The listing builds one solid part. Answer for the finished solid, in the listing's coordinates (mm). A direction names the side the tool comes from. Give positions to 0.01 mm unless a question says otherwise; leave off trailing zeros. Write each loop counter-clockwise with the first axis right and the second up, starting at its lowest first coordinate (ties: lowest second). Pieces come first, ordered by that corner, then holes. Notation, with made-up numbers: (43.5, -34) -> (69.5, -34) arc R17 ccw to (69.5, -9) -> close; hole circle Ø6 at (32, -17.5). An arc over 180 degrees is marked (long way). Write each question's results on one line, items separated by ' | '. Start each with the question number.
from build123d import *

# Parameters (mm, degrees)
BOSS_EXTRUDE1_DEPTH = 5
FILLET1_R           = 1
SKETCH2_R           = 1.5
CUT_EXTRUDE1_DEPTH  = 10


with BuildPart() as part:
    # Sketch1 → Boss-Extrude1 (new body, symmetric)
    with BuildSketch(Plane.XY):
        with BuildLine():
            Line((4, 0), (12, 0))
            Line((12, 0), (12, 1))
            Line((12, 1), (4.898979486, 1))
            ThreePointArc((4.898979486, 1), (0, 5), (-4.898979486, 1))
            Line((-4.898979486, 1), (-12, 1))
            Line((-12, 1), (-12, 0))
            Line((-12, 0), (-4, 0))
            ThreePointArc((-4, 0), (0, 4), (4, 0))
        make_face()
    extrude(amount=BOSS_EXTRUDE1_DEPTH, both=True)

    # Fillet1
    fillet1_edges = [part.edges().sort_by_distance(p)[0] for p in [
        (-12, 0.5, -5),
        (-12, 0.5, 5),
        (12, 0.5, 5),
        (12, 0.5, -5),
    ]]
    fillet(fillet1_edges, radius=FILLET1_R)

    # Sketch2 → Cut-Extrude1 (cut)
    with BuildSketch(Plane(origin=(0, 1, 0), x_dir=(1, 0, 0), z_dir=(0, 1, 0))):
        with Locations((-8, 0)):
            Circle(SKETCH2_R)
        with Locations((8, 0)):
            Circle(SKETCH2_R)
    extrude(amount=-CUT_EXTRUDE1_DEPTH, mode=Mode.SUBTRACT)


solid = part.part
1. Section C-C (z = -2) is taken. Write down the section's boundary in (x, y).
2. Section A-A (x = 8) is taken. Write down the section's boundary in (y, z), then the cut area to 3 significant figures.
3. A tool of negligible diameter and unlimited length cuts with its end or side. For faces 1 (the cylindrical face through (11.715, 0.507, -4.699)), 2 (the flat face through (-9.2, 1, 1.2)), from which of +Z, -Z, +X, -X, +Y, -Y can it reach the whole face along a straight path? Write none if from no direction.
4. Consider probe 1 along X at (y, z) = (0.6, 0); probe 2 along Z at (x, y) = (8, 0.3); probe 3 along Y at (x, z) = (6.5, -2.75). Determine where each line is inside the solid, lowest interval first. Write a range as [from, to].
5. Section B-B (y = 2.15) is taken. Write down the section's boundary in (x, z), then the cut area to 3 significant figures.
6. The mould has two halves that part along X. Classify faces 3 (the cylindrical face through (-9.5, 0.51, -0.07)), 4 (the flat face through (9.3, 1, 1.2)), 5 (the cylindrical face through (6.5, 0.51, -0.07)), 6 (the cylindrical face through (0, 5, 0)): pulls with the +X half, pulls with the -X half, needs draft (parallel to the pull), parting line crosses it, or undercut.
7. Section D-D (y = 0.6) is taken. Write down the section's boundary in (x, z), then the cut area to 3 significant figures.
8. Each of these flat-tipped pins is pushed along its axis until it touches: pin 1 Ø3 at (x, z) = (4, -1.5) entering from +Y; pin 2 Ø1 at (x, z) = (-6, 2.5) entering from -Y; pin 3 Ø3 at (x, z) = (5.5, 0.5) entering from +Y; pin 4 Ø1 at (y, z) = (3, -2.5) entering from -X. Where does it stop, or does it pass through?
Results:
1) outline: (-12, 0) -> (-4, 0) arc R4 cw to (4, 0) -> (12, 0) -> (12, 1) -> (4.9, 1) arc R5 ccw to (-4.9, 1) -> (-12, 1) -> close
2) outline: (0, -5) -> (1, -5) -> (1, -1.5) -> (0, -1.5) -> close; (0, 1.5) -> (1, 1.5) -> (1, 5) -> (0, 5) -> close | area: 7.00 mm²
3) face 1: -Z, +X, +Y, -Y | face 2: +Z, -Z, -X, +Y
4) probe 1: x = [-12, -9.5], [-6.5, -3.95], [3.95, 6.5], [9.5, 12] | probe 2: z = [-5, -1.5], [1.5, 5] | probe 3: y = [0, 1]
5) outline: (-4.51, -5) -> (-3.37, -5) -> (-3.37, 5) -> (-4.51, 5) -> close; (3.37, -5) -> (4.51, -5) -> (4.51, 5) -> (3.37, 5) -> close | area: 22.8 mm²
6) face 3: undercut | face 4: needs draft | face 5: undercut | face 6: parting line crosses it
7) outline: (-12, -4) arc R1 ccw to (-11, -5) -> (-3.95, -5) -> (-3.95, 5) -> (-11, 5) arc R1 ccw to (-12, 4) -> close; (3.95, -5) -> (11, -5) arc R1 ccw to (12, -4) -> (12, 4) arc R1 ccw to (11, 5) -> (3.95, 5) -> close; hole circle Ø3 at (-8, 0); hole circle Ø3 at (8, 0) | area: 146 mm²
8) pin 1: stops at y = 4.33 | pin 2: stops at y = 0 | pin 3: stops at y = 3 | pin 4: stops at x = -4.33
